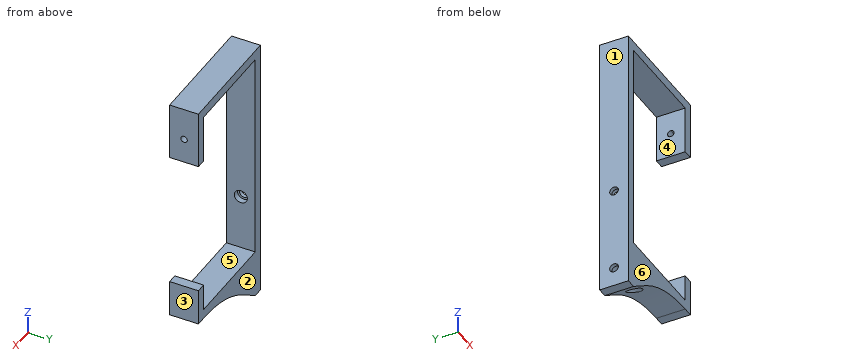
```python
from build123d import *

# Parameters (mm, degrees)
F1_W     = 5
F1_H     = 10
F1_W_2   = 50.2
F1_H_2   = 5
F1_H_3   = 11
F2_DEPTH = 15
F3_START = 25
F3_DEPTH = 49
F0_R     = 2.25
F4_DEPTH = 38.6
F5_START = 2
F0_R_2   = 3.4
F5_DEPTH = 47.7


with BuildPart() as f2:
    # F1 (on Front) → F2 (new body)
    with BuildSketch(Plane.XZ):
        Polygon((0, 34), (0, 0), (5, 0), (5, 5), (5, 34), align=None)
        with Locations((2.5, -5)):
            Rectangle(F1_W, F1_H)
        with Locations((30.1, 2.5)):
            Rectangle(F1_W_2, F1_H_2)
        with BuildLine():
            Line((55.2, 0), (5, 0))
            Line((5, 0), (5, -10))
            Line((5, -10), (5, -20))
            add(Edge.make_bspline(
                [(5, -20), (15.5953727663, -13.1017330475), (28.5827647895, 0), (55.2, 0)],
                knots=[0, 0, 0, 0, 54.0373944598, 54.0373944598, 54.0373944598, 54.0373944598], degree=3))
        make_face()
        Polygon((0, 120), (0, 34), (5, 34), (5, 115), (5, 120), align=None)
        with Locations((2.5, -15)):
            Rectangle(F1_W, F1_H)
        Polygon((55.2, 5), (55.2, 0), (60.2, 0), (60.2, 19), (55.2, 19), align=None)
        with Locations((30.1, 117.5)):
            Rectangle(F1_W_2, F1_H_2)
        Polygon((60.2, 120), (55.2, 120), (55.2, 115), (55.2, 101), (60.2, 101), align=None)
        with Locations((57.7, 95.5)):
            Rectangle(F1_W, F1_H_3)
    extrude(amount=F2_DEPTH)

    # F0 (on Right) → F3 (cut)
    with BuildSketch(Plane.YZ.offset(F3_START)):
        with BuildLine():
            ThreePointArc((-5.8, 103), (-6.297918472, 104.202081528), (-7.5, 104.7))
            ThreePointArc((-7.5, 104.7), (-8.702081528, 101.797918472), (-5.8, 103))
        make_face()
    extrude(amount=F3_DEPTH, mode=Mode.SUBTRACT)

    # F0 (on Right) → F4 (cut)
    with BuildSketch(Plane.YZ):
        with Locations((-7.5, 34)):
            Circle(F0_R)
        with Locations((-7.5, -10)):
            Circle(F0_R)
    extrude(amount=F4_DEPTH, mode=Mode.SUBTRACT)

    # F0 (on Right) → F5 (cut)
    with BuildSketch(Plane.YZ.offset(F5_START)):
        with Locations((-7.5, -10)):
            Circle(F0_R_2)
        with Locations((-7.5, -10)):
            Circle(F0_R, mode=Mode.SUBTRACT)
        with Locations((-7.5, 34)):
            Circle(F0_R_2)
        with Locations((-7.5, 34)):
            Circle(F0_R, mode=Mode.SUBTRACT)
    extrude(amount=F5_DEPTH, mode=Mode.SUBTRACT)


solid = f2.part
```
Build history of the part. All positions in model axes, mm. Face numbers are marked on the shaded views. A direction names the side the tool comes from. Give positions to 0.01 mm unless a question says otherwise; leave off trailing zeros. Loops run counter-clockwise (first coordinate to the right, second up) from the corner with the lowest first, then second, coordinate; pieces in that order, holes last. Notation, with made-up numbers: (44, 41) -> (97, 41) arc R21 cw to (97, 51) -> close; hole circle Ø1 at (-30, 13.25). An arc over 180 degrees is marked (long way). One line per question, with ' | ' between items.
Q1. Pull direction X, two halves, no side cores. Call the marked faces 1, 2, 3 and 4: pulls with the +X half, pulls with the -X half, needs draft (parallel to the pull), parting line crosses it, or undercut.
Filled sheet:
face 1: pulls with the -X half | face 2: needs draft | face 3: pulls with the +X half | face 4: undercut
Q2. Drill centre lines: line 1 along Z through (x, y) = (58.7, -7.5); line 2 along Z through (x, y) = (1.35, -7.5); line 3 along Z through (x, y) = (18.25, -7.5). Where is each one in solid material? Low to high. Write a range as [from, to].
Filled sheet:
line 1: z = [0, 19], [90, 101.3], [104.7, 120] | line 2: z = [-20, -12.25], [-7.75, 31.75], [36.25, 120] | line 3: z = [-6.6, 5], [115, 120]
Q3. Drop flat-ended pins along their axis: pin 1 (5 mm diameter, centred on y = -4.5, z = 81.5, fed in from -X); pin 2 (6 mm diameter, centred on y = -7.5, z = 34, fed in from +X); pin 3 (5 mm diameter, centred on x = 28, y = -10.5, fed in from -Z); pin 4 (4 mm diameter, centred on x = 57.5, y = -9, fed in from -Z). Give the stop position or say it passes through.
Filled sheet:
pin 1: stops at x = 0 | pin 2: stops at x = 2 | pin 3: stops at z = -6.7 | pin 4: stops at z = 0
Q4. Tool access for the marked faces 5 and 6: list every direction of +Z, -Z, +X, -X, +Y, -Y with a clear straight run to the whole face (end or side of a thin tool).
Filled sheet:
face 5: +Y, -Y | face 6: +Z, -Z, +X, -X, -Y
Q5. Cut at B-B, the plane z = 17.5. Write the cut outline in (x, y).
Filled sheet:
outline: (0, -15) -> (5, -15) -> (5, 0) -> (0, 0) -> close; (55.2, -15) -> (60.2, -15) -> (60.2, 0) -> (55.2, 0) -> close
Q6. Cut at C-C, the plane z = 34. Write the cut outline in (x, y).
Filled sheet:
outline: (0, -15) -> (5, -15) -> (5, -10.9) -> (2, -10.9) -> (2, -9.75) -> (0, -9.75) -> close; (0, -5.25) -> (2, -5.25) -> (2, -4.1) -> (5, -4.1) -> (5, 0) -> (0, 0) -> close
Q7. Cut at A-A, the plane x = 56.5. Write the cut outline in (y, z).
Filled sheet:
outline: (-15, 0) -> (0, 0) -> (0, 19) -> (-15, 19) -> close; (-15, 90) -> (0, 90) -> (0, 120) -> (-15, 120) -> close; hole circle Ø3.4 at (-7.5, 103)
Q8. Cut at D-D, the plane x = 9.5. Count the separate pieces of the cut face and the enclosed holes in it, plus the area to 3 significant figures.
Filled sheet:
separate pieces: 2 | enclosed holes: 1 | area: 367 mm²
